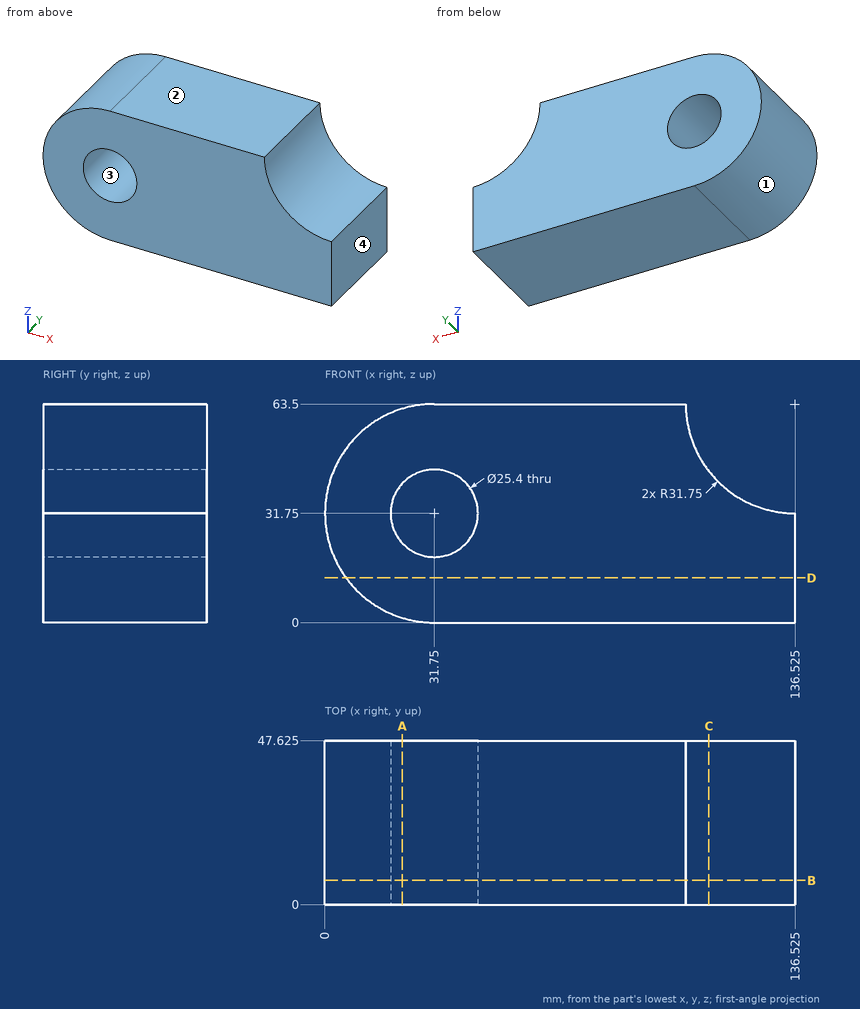
For this review, use the dimensioned drawing (mm, ordinates from the lowest corner) and the shaded views. Give positions to 0.01 mm unless a question says otherwise; leave off trailing zeros. Loops run counter-clockwise (first coordinate to the right, second up) from the corner with the lowest first, then second, coordinate; pieces in that order, holes last. Notation, with made-up numbers: (-39.5, 63) -> (3.5, 63) arc R25 cw to (3.5, 86) -> close; hole circle Ø11 at (-2, 35). An arc over 180 degrees is marked (long way). Use CSV: the item, a comma, the result in double quotes.
1. To check wall thickness, follow probe 1 along X at (y, z) = (13, 31) (3 decimals); probe 2 along Z at (x, y) = (31, 12); probe 3 along X at (y, z) = (29, 36.5). State the ranges of each line that lie inside material, in increasing order. Write a range as from..to.
Result:
probe 1,"x = 0.009..19.072, 44.428..136.525"
probe 2,"z = 0.01..19.07, 44.43..63.49"
probe 3,"x = 0.36..19.97, 43.53..119.82"
2. For P1, Ø20.5, axis at x = 31.75, z = 31.75, coming from the -Y side; P2, Ø1, axis at y = 19, z = 54, coming from the +X side; P3, Ø6, axis at y = 40, z = 44.5, coming from the +X side; P4, Ø10, axis at y = 23, z = 44, coming from the -X side, all flat-tipped, find the tip position at first contact; note any pin that passes through.
Result:
P1,"passes through"
P2,"stops at x = 106.39"
P3,"stops at x = 113.63"
P4,"stops at x = 0.84"
3. The part is to be moulded in two halves that separate along Z. For the marked faces 1, 2, 3 and 4, say which applies: +Z half, -Z half, draft (parallel to the pull), parting line (faces both ways), or undercut.
Result:
face 1,"parting line"
face 2,"+Z half"
face 3,"undercut"
face 4,"draft"
4. Consider section A-A, the plane x = 22.5. Write out the cut boundary in (y, z) (3 decimals).
Result:
outline,"(0, 1.377) -> (47.625, 1.377) -> (47.625, 23.048) -> (0, 23.048) -> close; (0, 40.452) -> (47.625, 40.452) -> (47.625, 62.123) -> (0, 62.123) -> close"
5. Consider section C-C, the plane x = 111.5. Write out the cut boundary in (y, z) (3 decimals).
Result:
outline,"(0, 0) -> (47.625, 0) -> (47.625, 43.96) -> (0, 43.96) -> close"
6. Consider section B-B, the plane y = 7. Write out the cut boundary in (x, z) (3 decimals), then the cut area to 3 significant figures.
Result:
outline,"(31.75, 0) -> (136.525, 0) -> (136.525, 31.75) arc R31.75 cw to (104.775, 63.5) -> (31.75, 63.5) arc R31.75 ccw to start; hole circle Ø25.4 at (31.75, 31.75)"
area,"6,940 mm²"
7. Consider section D-D, the plane z = 13. Write out the cut boundary in (x, y) (3 decimals).
Result:
outline,"(6.128, 0) -> (136.525, 0) -> (136.525, 47.625) -> (6.128, 47.625) -> close"
